Build history of the part. All positions in model axes, mm. A direction names the side the tool comes from. Round coordinates to 2 decimals unless told otherwise and drop trailing zeros. Write each loop counter-clockwise with the first axis right and the second up, starting at its lowest first coordinate (ties: lowest second). Pieces come first, ordered by that corner, then holes.
Item 1: 3-axis set-ups, long thin cutter, end or side, ignore diameter. For faces 1 (the flat face through (-45, -15, -1)), 2 (the flat face through (-1, -18, 50)), 3 (the flat face through (43.911, -15, 48)): which of +Z, -Z, +X, -X, +Y, -Y reach the whole face in a straight line?
Item 2: Band-saw the part on C-C, the plane x = -34. Write the cut outline in (y, z), then the cut area to 3 significant figures.
Item 3: Drop a flat-ended pin along its axis: pin 1 Ø2.5 at (x, z) = (9, 47.5) entering from +Y. Give the stop position or say it passes through.
Item 4: Band-saw the part on B-B, the plane z = -31.5. Write the cut outline in (x, y).
Item 5: Band-saw the part on A-A, the plane y = -21.25. Write the cut outline in (x, z), then the cut area to 3 significant figures.
Item 6: Wall check: probe 1 along Z at (x, y) = (-14, -4). Give the ranges that are in metal, low to high.
Item 7: Band-saw the part on D-D, the plane y = -15.75. Write the cut outline in (x, z), then the cut area to 3 significant figures.
Item 8: Mould opens along Y. For faces 4 (the flat face through (-4, -30, -48)), 5 (the flat face through (-50, -15, -1)), 6 (the flat face through (-43.911, -15, 48)), 7 (the flat face through (-4, 0, -48)) say: +Y half, -Y half, draft (parallel to the pull), parting line (faces both ways), or undercut.
```python
from build123d import *

# Parameters (mm, degrees)
F0_W     = 100
F0_H     = 100
F0_W_2   = 90
F0_H_2   = 90
F1_DEPTH = 30
F2_W     = 87.822602
F2_H     = 6.169355
F3_DEPTH = 25


with BuildPart() as f1:
    # F0 (on Front) → F1 (new body)
    with BuildSketch(Plane.XZ):
        Rectangle(F0_W, F0_H)
        Rectangle(F0_W_2, F0_H_2, mode=Mode.SUBTRACT)
    extrude(amount=F1_DEPTH)

    # F2 (on face) → F3 (cut)
    with BuildSketch(Plane.XY.offset(50)):
        with Locations((0, -14.697582)):
            Rectangle(F2_W, F2_H)
    extrude(amount=-F3_DEPTH, mode=Mode.SUBTRACT)


solid = f1.part
```
Results:
1. face 1: +Y, -Y
1. face 2: +Z, +X, -X, +Y, -Y
1. face 3: +Z
2. outline: (-30, -50) - (0, -50) - (0, -45) - (-30, -45) - close; (-30, 45) - (-17.78, 45) - (-17.78, 50) - (-30, 50) - close; (-11.61, 45) - (0, 45) - (0, 50) - (-11.61, 50) - close
2. area: 269 mm2
3. pin 1: stops at y = 0
4. outline: (-50, -30) - (-45, -30) - (-45, 0) - (-50, 0) - close; (45, -30) - (50, -30) - (50, 0) - (45, 0) - close
5. outline: (-50, -50) - (50, -50) - (50, 50) - (-50, 50) - close; hole (-45, -45) - (45, -45) - (45, 45) - (-45, 45) - close
5. area: 1,900 mm2
6. probe 1: z = -50 to -45, 45 to 50
7. outline: (-50, -50) - (50, -50) - (50, 50) - (43.91, 50) - (43.91, 45) - (45, 45) - (45, -45) - (-45, -45) - (-45, 45) - (-43.91, 45) - (-43.91, 50) - (-50, 50) - close
7. area: 1,460 mm2
8. face 4: -Y half
8. face 5: draft
8. face 6: undercut
8. face 7: +Y half
